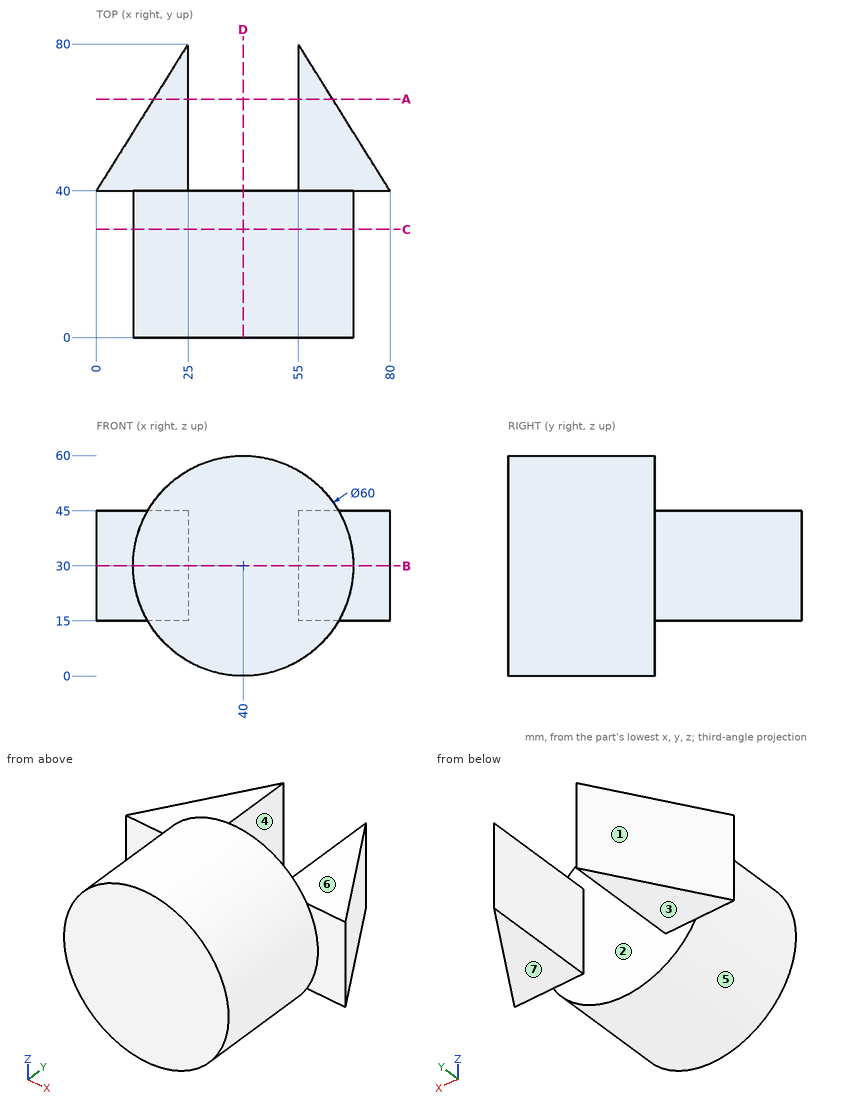
Design review of the part shown in the three views and the two pictorial views. Dimensions are in mm from the part's minimum x, y and z. A direction names the side the tool comes from. Round coordinates to 2 decimals unless told otherwise and drop trailing zeros. Write each loop counter-clockwise with the first axis right and the second up, starting at its lowest first coordinate (ties: lowest second). Pieces come first, ordered by that corner, then holes.
1) Insertion check: pin 1 Ø2 at (x, y) = (33, 23) entering from -Z; pin 2 Ø5 at (x, z) = (8.5, 32) entering from -Y; pin 3 Ø12.5 at (x, y) = (10, 60.5) entering from +Z; pin 4 Ø24 at (y, z) = (66.5, 25.5) entering from -X. Each pin has a flat end and moves straight along its axis. Give the tip position at first contact, or say it passes through.
Answer below:
pin 1: stops at z = 0.61
pin 2: stops at y = 0
pin 3: stops at z = 45
pin 4: stops at x = 9.06
2) Take a section at B-B on z = 30. Give the boundary of the cut face in (x, y).
Answer below:
outline: (0, 40) - (10, 40) - (10, 0) - (70, 0) - (70, 40) - (80, 40) - (55, 80) - (55, 40) - (25, 40) - (25, 80) - close
3) Take a section at C-C on y = 29.5. Give the boundary of the cut face in (x, z), then the cut area to 3 significant figures.
Answer below:
outline: circle Ø60 at (40, 30)
area: 2,830 mm2
4) Take a section at D-D on x = 40. Give the boundary of the cut face in (y, z).
Answer below:
outline: (0, 0) - (40, 0) - (40, 60) - (0, 60) - close
5) Mouldability with a two-part tool opening along X and no side actions: class the marked faces 1, 2 and 3 as +X half, -X half, draft (parallel to the pull), parting line (faces both ways), or undercut.
Answer below:
face 1: -X half
face 2: undercut
face 3: draft
6) Take a section at A-A on y = 65. Give the boundary of the cut face in (x, z) (3 decimals).
Answer below:
outline: (15.625, 15) - (25, 15) - (25, 45) - (15.625, 45) - close; (55, 15) - (64.375, 15) - (64.375, 45) - (55, 45) - close
7) Machinability: for the marked faces 4, 5, 6 and 7, which of the approach directions +Z, -Z, +X, -X, +Y, -Y give a long, thin tool a straight path to every point of the face, cutting with its end or side? Answer none if there is none.
Answer below:
face 4: +Z, -Z, +Y
face 5: -Y
face 6: +Z, +X, -X, +Y
face 7: -Z, +X, -X, +Y
8) For line 1 along Z through (x, y) = (66, 57); line 2 along Y through (x, z) = (12.5, 38.5); line 3 along Y through (x, z) = (36.5, 41.5), list the stretches that pass through material, from the lowest coordinate up.
Answer below:
line 1: z = 15 to 45
line 2: y = 0 to 60
line 3: y = 0 to 40
